Work out the finished part from the listing and answer in its coordinate system (mm). A direction names the side the tool comes from. Round coordinates to 2 decimals unless told otherwise and drop trailing zeros. Loops run counter-clockwise (first coordinate to the right, second up) from the corner with the lowest first, then second, coordinate; pieces in that order, holes last. Notation, with made-up numbers: (-5.75, -12) -> (43.25, -12) arc R35 ccw to (43.25, 21) -> close; hole circle Ø3 at (80.5, 10.5). An arc over 180 degrees is marked (long way). Use one line per item in the form item = value.
```python
from build123d import *

# Parameters (mm, degrees)
F0_W         = 24.6
F0_H         = 29.5
F0_W_2       = 16.6
F0_H_2       = 25.5
F1_DEPTH     = 270
F2_R         = 1.99999
F3_T1_DEPTH  = 280
F3_T4_ANGLE  = 90
F3_T6_ANGLE  = 90
F3_T8_ANGLE  = 90
F3_T10_ANGLE = 90


# Not quite as in the source:
# - a fillet or chamfer that OpenCascade refuses, or shapes differently, is made with other operations: its cross-section is extruded or revolved along the edge and cut away or added
# - a fillet or chamfer is up to 0.001 mm smaller than in the source, because OpenCascade refuses the exact size


with BuildPart() as f1:
    # F0 (on Top) → F1 (new body)
    with BuildSketch(Plane.XY):
        Rectangle(F0_W, F0_H)
        Rectangle(F0_W_2, F0_H_2, mode=Mode.SUBTRACT)
    extrude(amount=-F1_DEPTH)

    # F2 (radius 2 in the source; OpenCascade refuses exactly that, so slightly less here)
    f2_edges = [f1.edges().sort_by_distance(p)[0] for p in [
        (-12.3, 0, -270),
        (0, 14.75, -270),
        (12.3, 0, -270),
        (0, -14.75, -270),
    ]]
    fillet(f2_edges, radius=F2_R)

    # F3: fillet of radius 4 on 4 edges, made by hand

    # F3_s2 → F3_t1 (cut)
    with BuildSketch(Plane.XY.offset(-270)):
        with BuildLine():
            ThreePointArc((8.3, 14.75), (11.1284271247, 13.5784271247), (12.3, 10.75))
            Line((12.3, 10.75), (12.3, 14.75))
            Line((12.3, 14.75), (8.3, 14.75))
        make_face()
        with BuildLine():
            ThreePointArc((-12.3, 10.75), (-11.1284271247, 13.5784271247), (-8.3, 14.75))
            Line((-8.3, 14.75), (-12.3, 14.75))
            Line((-12.3, 14.75), (-12.3, 10.75))
        make_face()
        with BuildLine():
            ThreePointArc((8.3, -14.75), (11.1284271247, -13.5784271247), (12.3, -10.75))
            Line((12.3, -10.75), (12.3, -14.75))
            Line((12.3, -14.75), (8.3, -14.75))
        make_face()
        with BuildLine():
            ThreePointArc((-12.3, -10.75), (-11.1284271247, -13.5784271247), (-8.3, -14.75))
            Line((-8.3, -14.75), (-12.3, -14.75))
            Line((-12.3, -14.75), (-12.3, -10.75))
        make_face()
    extrude(amount=F3_T1_DEPTH, mode=Mode.SUBTRACT)

    # F3_s3 → F3_t4 (revolve, cut)
    with BuildSketch(Plane.YZ.offset(-8.3)):
        with BuildLine():
            ThreePointArc((-12.75001, -270), (-14.1642164913, -269.4142164913), (-14.75, -268.00001))
            Line((-14.75, -268.00001), (-14.75, -270))
            Line((-14.75, -270), (-12.75001, -270))
        make_face()
    revolve(axis=Axis((-8.3, -10.75, -270), (0, 0, -1)), revolution_arc=F3_T4_ANGLE, mode=Mode.SUBTRACT)

    # F3_s5 → F3_t6 (revolve, cut)
    with BuildSketch(Plane.XZ.offset(10.75)):
        with BuildLine():
            ThreePointArc((10.30001, -270), (11.7142164913, -269.4142164913), (12.3, -268.00001))
            Line((12.3, -268.00001), (12.3, -270))
            Line((12.3, -270), (10.30001, -270))
        make_face()
    revolve(axis=Axis((8.3, -10.75, -270), (0, 0, -1)), revolution_arc=F3_T6_ANGLE, mode=Mode.SUBTRACT)

    # F3_s7 → F3_t8 (revolve, cut)
    with BuildSketch(Plane.XZ.offset(-10.75)):
        with BuildLine():
            ThreePointArc((-10.30001, -270), (-11.7142164913, -269.4142164913), (-12.3, -268.00001))
            Line((-12.3, -268.00001), (-12.3, -270))
            Line((-12.3, -270), (-10.30001, -270))
        make_face()
    revolve(axis=Axis((-8.3, 10.75, -270), (0, 0, -1)), revolution_arc=F3_T8_ANGLE, mode=Mode.SUBTRACT)

    # F3_s9 → F3_t10 (revolve, cut)
    with BuildSketch(Plane.YZ.offset(8.3)):
        with BuildLine():
            ThreePointArc((12.75001, -270), (14.1642164913, -269.4142164913), (14.75, -268.00001))
            Line((14.75, -268.00001), (14.75, -270))
            Line((14.75, -270), (12.75001, -270))
        make_face()
    revolve(axis=Axis((8.3, 10.75, -270), (0, 0, -1)), revolution_arc=F3_T10_ANGLE, mode=Mode.SUBTRACT)


solid = f1.part
```
(1) Find section C-C, the plane z = -71. Write down the section's boundary in (x, y).
Completed:
outline = (-12.3, -10.75) arc R4 ccw to (-8.3, -14.75) -> (8.3, -14.75) arc R4 ccw to (12.3, -10.75) -> (12.3, 10.75) arc R4 ccw to (8.3, 14.75) -> (-8.3, 14.75) arc R4 ccw to (-12.3, 10.75) -> close; hole (-8.3, -12.75) -> (8.3, -12.75) -> (8.3, 12.75) -> (-8.3, 12.75) -> close
(2) For faces 1 (the flat face through (0, -14.75, -132)), 2 (the flat face through (-8.3, 0, -133)), determine the directions among +Z, -Z, +X, -X, +Y, -Y from which every point of the face is accessible in a straight line to the end or side of a thin tool.
Completed:
face_1 = +Z, -Z, +X, -X, -Y
face_2 = +Z, -Z
(3) Find section B-B, the plane y = 0.75. Write down the section's boundary in (x, z), then the cut area to 3 significant figures.
Completed:
outline = (-12.3, -268) arc R2 ccw to (-10.3, -270) -> (-8.3, -270) -> (-8.3, 0) -> (-12.3, 0) -> close; (8.3, -270) -> (10.3, -270) arc R2 ccw to (12.3, -268) -> (12.3, 0) -> (8.3, 0) -> close
area = 2,160 mm2
(4) Consider L1, parallel to X at y = -11.25, z = -248; L2, parallel to Y at x = 3.25, z = -207.5. Determine where each line is inside the solid, lowest interval first.
Completed:
L1 = -12.27 to -8.3, 8.3 to 12.27
L2 = -14.75 to -12.75, 12.75 to 14.75
(5) For a pull along Y with two mould halves and no side action, classify faces 3 (the flat face through (0, 14.75, -132)), 4 (the flat face through (0, -12.75, -133)), 5 (the flat face through (-11, 0, 0)) as +Y half, -Y half, draft (parallel to the pull), parting line (faces both ways), or undercut.
Completed:
face_3 = +Y half
face_4 = undercut
face_5 = draft
